```python
from build123d import *

# Parameters (mm, degrees)
F0_W     = 50.8
F0_H     = 57.15
F1_DEPTH = 63.5
F3_D     = 6.35
F3_DEPTH = 12.7
F3_TIP   = 1.9077324654
F4_R     = 6.35


with BuildPart() as f1:
    # F0 (on Front) → F1 (new body)
    with BuildSketch(Plane.XZ):
        with Locations((25.4, 28.575)):
            Rectangle(F0_W, F0_H)
    extrude(amount=F1_DEPTH)

    # F3
    with Locations(Plane.XY.offset(57.15)):
        with Locations((20.8245180547, -28.2227080315)):
            Hole(F3_D / 2, depth=F3_DEPTH)
            with Locations((0, 0, -(F3_DEPTH + F3_TIP / 2))):  # 118° drill point
                Cone(0, F3_D / 2, F3_TIP, mode=Mode.SUBTRACT)

    # F4
    f4_edges = [f1.edges().sort_by_distance(p)[0] for p in [
        (50.8, -31.75, 0),
        (50.8, -31.75, 57.15),
        (50.8, 0, 28.575),
        (50.8, -63.5, 28.575),
        (0, -63.5, 28.575),
        (25.4, -63.5, 0),
        (25.4, -63.5, 57.15),
        (25.4, 0, 57.15),
        (0, -31.75, 57.15),
        (0, 0, 28.575),
        (25.4, 0, 0),
        (0, -31.75, 0),
    ]]
    fillet(f4_edges, radius=F4_R)


solid = f1.part
```
CAD build for the part. Positions are in the model's coordinates, mm. Give positions to 0.01 mm unless a question says otherwise; leave off trailing zeros. Order: outer loops, then holes, each group sorted by start corner. A loop starts at its lowest first (then second) coordinate and runs counter-clockwise, first axis right, second up. Notation, with made-up numbers: M 3.25,27 L 33.25,27 A22 ccw 33.25,64 Z; hole C -30,12 d11. An arc over 180 degrees is marked long. Put each result on its own line as item: value. Start each with the question number.
(1) Saw through at A-A, the plane z = 46. Write the cut outline in (x, y) (3 decimals), then the cut area to 3 significant figures.
(2) Saw through at B-B, the plane x = 47. Write the cut outline in (y, z).
(3) Saw through at C-C, the plane y = -5.5. Write the cut outline in (x, z).
(4) Drill centre lines: line 1 along X through (y, z) = (-28, 47); line 2 along Z through (x, y) = (6, -41); line 3 along Y through (x, z) = (21, 52.5). Where is each one in solid material? Low to high.
(5) Mould opens along Y. For faces 1 (the cylindrical face through (48.89, -32.11, 1.81)), 2 (the conical face through (21.33, -28.43, 42.87)), 3 (the cylindrical face through (48.89, -61.69, 28.89)), 4 (the cylindrical face through (19.36, -31.04, 50.71)) say: +Y half, -Y half, draft (parallel to the pull), parting line (faces both ways), or undercut.
Check result:
1. outline: M 0,-57.15 A6.35 ccw 6.35,-63.5 L 44.45,-63.5 A6.35 ccw 50.8,-57.15 L 50.8,-6.35 A6.35 ccw 44.45,0 L 6.35,0 A6.35 ccw 0,-6.35 Z; hole C 20.825,-28.223 d6.35
1. area: 3,160 mm2
2. outline: M -62.97,6.35 A5.82 ccw -57.15,0.53 L -6.35,0.53 A5.82 ccw -0.53,6.35 L -0.53,50.8 A5.82 ccw -6.35,56.62 L -57.15,56.62 A5.82 ccw -62.97,50.8 Z
3. outline: M 0.06,6.35 A6.29 ccw 6.35,0.06 L 44.45,0.06 A6.29 ccw 50.74,6.35 L 50.74,50.8 A6.29 ccw 44.45,57.09 L 6.35,57.09 A6.29 ccw 0.06,50.8 Z
4. line 1: x = 0 to 17.66, 23.99 to 50.8
4. line 2: z = 0.01 to 57.14
4. line 3: y = -63.27 to -31.39, -25.05 to -0.23
5. face 1: draft
5. face 2: undercut
5. face 3: -Y half
5. face 4: undercut
